```python
from build123d import *

# Parameters (mm, degrees)
SKETCH1_R           = 12.5
BOSS_EXTRUDE1_DEPTH = 17.5
SKETCH2_R           = 2
BOSS_EXTRUDE2_DEPTH = 26
CHAMFER1_SIZE       = 10
SKETCH3_W           = 28.997372317
SKETCH3_H           = 7.197339184
CUT_EXTRUDE1_DEPTH  = 20
SKETCH4_R           = 5
CUT_EXTRUDE2_DEPTH  = 5
SKETCH5_R           = 3.5
BOSS_EXTRUDE3_DEPTH = 3.5
CUT_EXTRUDE6_START  = -1
CUT_EXTRUDE6_DEPTH  = 1
SKETCH11_R          = 5
SKETCH11_R_2        = 1.25
BOSS_EXTRUDE4_DEPTH = 5
SKETCH12_R          = 2.5
CUT_EXTRUDE7_DEPTH  = 5


with BuildPart() as part:
    # Sketch1 → Boss-Extrude1 (new, symmetric)
    with BuildSketch(Plane(origin=(0, 0, 0), x_dir=(0, 0, -1), z_dir=(1, 0, 0))):
        Circle(SKETCH1_R)
    extrude(amount=BOSS_EXTRUDE1_DEPTH, both=True)

    # Sketch2 → Boss-Extrude2 (add, symmetric)
    with BuildSketch(Plane(origin=(0, 0, 0), x_dir=(0, 0, -1), z_dir=(1, 0, 0))):
        with Locations(Location((0, 0, 0), (0, 0, 180))):
            Circle(SKETCH2_R)
    extrude(amount=BOSS_EXTRUDE2_DEPTH, both=True)

    # Chamfer1
    chamfer1_edges = [part.edges().sort_by_distance(p)[0] for p in [
        (-17.5, 0, 12.5),
        (17.5, 0, 12.5),
    ]]
    chamfer(chamfer1_edges, length=CHAMFER1_SIZE)

    # Sketch3 → Cut-Extrude1 (cut, symmetric)
    with BuildSketch(Plane(origin=(0, 0, 0), x_dir=(0, 0, -1), z_dir=(1, 0, 0))):
        with Locations((0.644848308, -13.770631617)):
            Rectangle(SKETCH3_W, SKETCH3_H)
    extrude(amount=CUT_EXTRUDE1_DEPTH, both=True, mode=Mode.SUBTRACT)

    # Sketch4 → Cut-Extrude2 (cut)
    with BuildSketch(Plane.XZ.offset(10.171962025)):
        with Locations(Location((0, 0, 0), (0, 0, 270))):
            Circle(SKETCH4_R)
    extrude(amount=-CUT_EXTRUDE2_DEPTH, mode=Mode.SUBTRACT)

    # Sketch5 → Boss-Extrude3 (add)
    with BuildSketch(Plane.ZY.offset(26)):
        Circle(SKETCH5_R)
    boss_extrude3 = extrude(amount=BOSS_EXTRUDE3_DEPTH)

    # Sketch6 → Cut-Extrude6 (cut)
    with BuildSketch(Plane.ZY.offset(29.5).offset(CUT_EXTRUDE6_START)):
        with BuildLine():
            Line((2.803043133, -2.095936352), (-2.095936352, 2.803043133))
            ThreePointArc((-2.095936352, 2.803043133), (-2.474873734, 2.474873734), (-2.803043133, 2.095936352))
            Line((-2.803043133, 2.095936352), (2.095936352, -2.803043133))
            ThreePointArc((2.095936352, -2.803043133), (2.474873734, -2.474873734), (2.803043133, -2.095936352))
        make_face()
    cut_extrude6 = extrude(amount=CUT_EXTRUDE6_DEPTH, mode=Mode.SUBTRACT)

    # Mirror1: Boss-Extrude3, Cut-Extrude6 across plane
    add(boss_extrude3.mirror(Plane(origin=(0, 0, 0), x_dir=(0, 0, 1), z_dir=(1, 0, 0))))
    add(cut_extrude6.mirror(Plane(origin=(0, 0, 0), x_dir=(0, 0, 1), z_dir=(1, 0, 0))), mode=Mode.SUBTRACT)

    # Sketch11 → Boss-Extrude4 (add)
    with BuildSketch(Plane.XZ.offset(10.171962025)):
        Circle(SKETCH11_R)
        with Locations(Location((0, 0, 0), (0, 0, 270))):
            Circle(SKETCH11_R_2, mode=Mode.SUBTRACT)
    extrude(amount=-BOSS_EXTRUDE4_DEPTH)

    # Sketch12 → Cut-Extrude7 (cut)
    with BuildSketch(Plane.XZ.offset(10.171962025)):
        with Locations(Location((0, 0, 0), (0, 0, 270))):
            Circle(SKETCH12_R)
    extrude(amount=-CUT_EXTRUDE7_DEPTH, mode=Mode.SUBTRACT)


solid = part.part
```
The listing builds one solid part. Answer for the finished solid, in the listing's coordinates (mm). A direction names the side the tool comes from. Give positions to 0.01 mm unless a question says otherwise; leave off trailing zeros. Order: outer loops, then holes, each group sorted by start corner. A loop starts at its lowest first (then second) coordinate and runs counter-clockwise, first axis right, second up.
Item 1: The part is cut by section D-D, the plane x = 11. Give the vertices of the cut face in (y, z), and give its area (3 significant figures).
From the geometry:
outline: circle Ø18 at (0, 0)
area: 254 mm2
Item 2: The part is cut by section C-C, the plane x = -16. Give the vertices of the cut face in (y, z).
From the geometry:
outline: circle Ø8 at (0, 0)
Item 3: Given pin 1 Ø8 at (x, z) = (-1.5, 8.5) entering from +Y; pin 2 Ø4 at (x, z) = (8.5, 6.5) entering from -Y; pin 3 Ø12 at (x, y) = (-19.5, -2) entering from +Z; pin 4 Ø1 at (x, y) = (-6.5, 9) entering from -Z, each flat-ended and moving along its own axis, determine where each tip first touches the part or whether it passes through.
From the geometry:
pin 1: stops at y = 11.66
pin 2: stops at y = -10.17
pin 3: stops at z = 6.34
pin 4: stops at z = -9.17
Item 4: For a pull along X with two mould halves and no side action, classify faces 1 (the face through (-22, 2, 0)), 2 (the face through (29.5, 1, 1)), 3 (the face through (0.105, 12.492, -0.441)) as pulls with the +X half, pulls with the -X half, needs draft (parallel to the pull), parting line crosses it, or undercut.
From the geometry:
face 1: undercut
face 2: pulls with the +X half
face 3: needs draft
Item 5: The part is cut by section A-A, the plane x = 0. Give the vertices of the cut face in (y, z), and give its area (3 significant figures).
From the geometry:
outline: (-10.17, -7.27) arc R12.5 ccw (long way) to (-10.17, 7.27) - (-10.17, 2.5) - (-5.17, 2.5) - (-5.17, -2.5) - (-10.17, -2.5) - close
area: 443 mm2
Item 6: Find the intervals of material crossed by probe 1 along X at (y, z) = (-6.2, 0); probe 2 along X at (y, z) = (-7.8, 0); probe 3 along X at (y, z) = (-7.75, 7.5), in increasing order.
From the geometry:
probe 1: x = -13.8 to -2.5, 2.5 to 13.8
probe 2: x = -12.2 to -2.5, 2.5 to 12.2
probe 3: x = -9.22 to 9.22
Item 7: Which of the six approach directions +Z, -Z, +X, -X, +Y, -Y give full straight-line access (tool end or side, diameter ignored) to faces 4 (the face through (-28.5, 0, 0)), 5 (the face through (-26, -2, 2)), 6 (the face through (28.993, 0.319, 0.388))?
From the geometry:
face 4: -X
face 5: none
face 6: +X
